The model under review builds one solid part; all positions refer to its coordinate system, in mm. A direction names the side the tool comes from. Coordinates: 2 decimals unless noted, no trailing zeros. Order: outer loops, then holes, each group sorted by start corner. A loop starts at its lowest first (then second) coordinate and runs counter-clockwise, first axis right, second up. Notation, with made-up numbers: (65.25, 51.25) -> (72.25, 51.25) arc R19 ccw to (72.25, 61.25) -> close; hole circle Ø3 at (9.25, -13). An arc over 180 degrees is marked (long way). Put each result on its own line as item: value.
from build123d import *

# Parameters (mm, degrees)
CROQUIS1_W              = 37
CROQUIS1_H              = 23.3
SALIENTE_EXTRUIR1_DEPTH = 250
CROQUIS2_W              = 32
CROQUIS2_H              = 20.8
CORTAR_EXTRUIR1_DEPTH   = 250
CROQUIS3_R              = 1.25
CORTAR_EXTRUIR2_DEPTH   = 250


with BuildPart() as part:
    # Croquis1 → Saliente-Extruir1 (new body)
    with BuildSketch(Plane(origin=(0, 0, 0), x_dir=(1, 0, 0), z_dir=(0, 1, 0))):
        Rectangle(CROQUIS1_W, CROQUIS1_H)
    extrude(amount=SALIENTE_EXTRUIR1_DEPTH)

    # Croquis2 → Cortar-Extruir1 (cut)
    with BuildSketch(Plane(origin=(0, 250, 0), x_dir=(1, 0, 0), z_dir=(0, 1, 0))):
        with Locations((0, 1.25)):
            Rectangle(CROQUIS2_W, CROQUIS2_H)
    extrude(amount=-CORTAR_EXTRUIR1_DEPTH, mode=Mode.SUBTRACT)

    # Croquis3 → Cortar-Extruir2 (cut)
    with BuildSketch(Plane.XY.offset(11.65)):
        with Locations((0, 212)):
            Circle(CROQUIS3_R)
    extrude(amount=-CORTAR_EXTRUIR2_DEPTH, mode=Mode.SUBTRACT)


solid = part.part
Item 1: Consider section B-B on y = 122. Write out the cut boundary in (x, z).
Answers below:
outline: (-18.5, -11.65) -> (-16, -11.65) -> (-16, 9.15) -> (16, 9.15) -> (16, -11.65) -> (18.5, -11.65) -> (18.5, 11.65) -> (-18.5, 11.65) -> close
Item 2: Consider section A-A on z = -4.25. Write out the cut boundary in (x, y), and give its area (3 significant figures).
Answers below:
outline: (-18.5, 0) -> (-16, 0) -> (-16, 250) -> (-18.5, 250) -> close; (16, 0) -> (18.5, 0) -> (18.5, 250) -> (16, 250) -> close
area: 1,250 mm^2
Item 3: Mouldability with a two-part tool opening along X and no side actions: class faces 3 (the flat face through (16, 127, -1)), 4 (the flat face through (1.3, 250, 9.4)), 5 (the flat face through (18.5, 123, 0)) as +X half, -X half, draft (parallel to the pull), parting line (faces both ways), or undercut.
Answers below:
face 3: undercut
face 4: draft
face 5: +X half
Item 4: Consider section C-C on x = 5.5. Write out the cut boundary in (y, z).
Answers below:
outline: (0, 9.15) -> (250, 9.15) -> (250, 11.65) -> (0, 11.65) -> close
Item 5: For line 1 (X direction, y = 214.5, z = 6); line 2 (X direction, y = 212, z = 9.7); line 3 (Y direction, x = 0, z = 9.7), list the stretches that pass through material, from the lowest coordinate up. Write a range as from..to.
Answers below:
line 1: -18.5..-16, 16..18.5
line 2: -18.5..-1.25, 1.25..18.5
line 3: 0..210.75, 213.25..250
Item 6: For faces 1 (the flat face through (0, 123, 11.65)), 2 (the flat face through (0, 127, 9.15)), list the 3-axis set-ups (+Z, -Z, +X, -X, +Y, -Y) from which the entire face can be reached by the end or side of a thin tool; tool diameter is ignored.
Answers below:
face 1: +Z, +X, -X, +Y, -Y
face 2: -Z, +Y, -Y
Item 7: For pin 1 Ø3 at (x, y) = (0, 212) entering from -Z; pin 2 Ø3 at (x, z) = (-0.5, 7) entering from +Y, all flat-tipped, find the tip position at first contact; note any pin that passes through.
Answers below:
pin 1: z = 9.15
pin 2: through
